from build123d import *

# Parameters (mm, degrees)
SKETCH1_R           = 66.675
SKETCH1_R_2         = 15
BOSS_EXTRUDE1_DEPTH = 57
SKETCH2_R           = 73.25
SKETCH2_R_2         = 66.675
BOSS_EXTRUDE2_DEPTH = 9
LPATTERN1_COUNT     = 3
LPATTERN1_PITCH     = 21


with BuildPart() as part:
    # Sketch1 → Boss-Extrude1 (new body)
    with BuildSketch(Plane.XY):
        Circle(SKETCH1_R)
        Circle(SKETCH1_R_2, mode=Mode.SUBTRACT)
    extrude(amount=-BOSS_EXTRUDE1_DEPTH)

    # Sketch2 → Boss-Extrude2 (add)
    with BuildSketch(Plane.XY.offset(-3)):
        Circle(SKETCH2_R)
        Circle(SKETCH2_R_2, mode=Mode.SUBTRACT)
    boss_extrude2 = extrude(amount=-BOSS_EXTRUDE2_DEPTH)

    # LPattern1: Boss-Extrude2 ×3
    with Locations(*[(0, 0, -i * LPATTERN1_PITCH) for i in range(1, LPATTERN1_COUNT)]):
        add(boss_extrude2)


solid = part.part
Read the model definition and answer for the solid it produces. Units are mm, in the model's axes. A direction names the side the tool comes from. Give positions to 0.01 mm unless a question says otherwise; leave off trailing zeros. Loops run counter-clockwise (first coordinate to the right, second up) from the corner with the lowest first, then second, coordinate; pieces in that order, holes last. Notation, with made-up numbers: (45.25, 38) - (59.25, 38) arc R19 cw to (59.25, 60) - close; hole circle Ø1 at (-33, 60.25). An arc over 180 degrees is marked (long way). Answer as CSV lines item,"result". Start each with the question number.
1) Find section C-C (y = -42). Write down the section's boundary in (x, z).
2) Which of the six approach directions +Z, -Z, +X, -X, +Y, -Y give full straight-line access (tool end or side, diameter ignored) to faces 1 (the face through (16, -65, -12)), 2 (the face through (-16, 1, -57)), 3 (the face through (63.596, 20.027, -1.479)), 4 (the face through (63.596, 20.027, -55.479))?
3) Determine the mould class of faces 5 (the face through (-15.88, -71.51, -7.44)), 6 (the face through (-16, 1, 0)), 7 (the face through (16, -65, -45)) for opening direction Z: released by +Z, released by -Z, zero draft, split by the parting line, or undercut.
4) Find section D-D (x = 36). Write down the section's boundary in (y, z).
5) Each of these flat-tipped pins is pushed along its axis until it touches: pin 1 Ø12 at (y, z) = (19, -24.5) entering from -X; pin 2 Ø12 at (x, z) = (-27, -38) entering from -Y; pin 3 Ø2 at (x, z) = (-50, -45.5) entering from -Y. Where does it stop, or does it pass through?
6) Straight lines are drawn through the part: L1, parallel to Z at x = -54.5, y = 43; L2, parallel to Y at x = 0, z = -32; L3, parallel to Y at x = 0, z = -36 (3 decimals). For each, find the intervals that lie inside material, in ascending order. Write a range as from..to.
Findings below:
1,outline,"(-60.01, -54) - (-51.78, -54) - (-51.78, -57) - (51.78, -57) - (51.78, -54) - (60.01, -54) - (60.01, -45) - (51.78, -45) - (51.78, -33) - (60.01, -33) - (60.01, -24) - (51.78, -24) - (51.78, -12) - (60.01, -12) - (60.01, -3) - (51.78, -3) - (51.78, 0) - (-51.78, 0) - (-51.78, -3) - (-60.01, -3) - (-60.01, -12) - (-51.78, -12) - (-51.78, -24) - (-60.01, -24) - (-60.01, -33) - (-51.78, -33) - (-51.78, -45) - (-60.01, -45) - close"
2,face 1,"none"
2,face 2,"-Z, +X, -X, +Y, -Y"
2,face 3,"+Z"
2,face 4,"-Z"
3,face 5,"zero draft"
3,face 6,"released by +Z"
3,face 7,"undercut"
4,outline,"(-63.79, -54) - (-56.12, -54) - (-56.12, -57) - (56.12, -57) - (56.12, -54) - (63.79, -54) - (63.79, -45) - (56.12, -45) - (56.12, -33) - (63.79, -33) - (63.79, -24) - (56.12, -24) - (56.12, -12) - (63.79, -12) - (63.79, -3) - (56.12, -3) - (56.12, 0) - (-56.12, 0) - (-56.12, -3) - (-63.79, -3) - (-63.79, -12) - (-56.12, -12) - (-56.12, -24) - (-63.79, -24) - (-63.79, -33) - (-56.12, -33) - (-56.12, -45) - (-63.79, -45) - close"
5,pin 1,"x = -72.09"
5,pin 2,"y = -69.32"
5,pin 3,"y = -54.45"
6,L1,"-54..-45, -33..-24, -12..-3"
6,L2,"-73.25..-15, 15..73.25"
6,L3,"-66.675..-15, 15..66.675"
